```python
from build123d import *

# Parameters (mm, degrees)
F1_W            = 3.9823013358
F1_H            = 8.4623899311
F3_ANGLE_BACK   = 15
F3_ANGLE        = 30
F3_COPIES_COUNT = 4
F5_ANGLE_BACK   = 15
F5_ANGLE        = 30
F5_COPIES_COUNT = 4


# Not quite as in the source:
# - a pattern or mirror of a feature is missing from the dataset's text; its kind, count and spacing are read off the source's solid


with BuildPart() as f2:
    # F0 (on Front) → F2 (revolve)
    with BuildSketch(Plane.XZ):
        Polygon((0, 57.2826008411), (0, -18.7173991589), (18, -18.7173991589), (12.58260943, -15.5477793887), (8.3016352728, -13.0588412285), (8.3016352728, -4.7955662012), (8.3016352728, 1.6756732948), (8.3016352728, 5.1601859741), (9.1348709539, 7.4490089901), (10.7923932374, 10.6456615031), (10.7923932374, 16.8021768332), (8.3016352728, 20.8275895566), (8.3016352728, 28.1680505723), (9.7421156242, 29.4479895383), (8.7946596922, 30.5142838619), (9.8650568815, 31.4653853958), (8.8950488368, 32.5570605196), (9.914630721, 33.4630101088), (8.9067585183, 34.5972986517), (9.9263404025, 35.5032482409), (8.9067585183, 36.6507151981), (12.6114161685, 41.0112217069), (12.6114161685, 42.9367274046), (8.3016352728, 42.9367274046), (12.4439811334, 47.2063235939), (5.8302935213, 43.1041605771), (5.8302935213, 49.299262464), align=None)
    revolve(axis=Axis((0, 0, 19.2826008411), (0, 0, -1)))

    # F1 (on Front) → F3 (revolve)
    with BuildSketch(Plane.XZ, mode=Mode.PRIVATE) as f3_sk:
        with Locations((9.1009729076, 32.2875799611)):
            Rectangle(F1_W, F1_H)
    f3 = revolve(f3_sk.sketch.rotate(Axis((0, 0, 30.8512914926), (0, 0, -1)), -F3_ANGLE_BACK), axis=Axis((0, 0, 30.8512914926), (0, 0, -1)), revolution_arc=F3_ANGLE)

    # F3_copies: F3 ×4 about axis
    f3_copies_axis = Axis((0, 0, 0), (0, 0, 1))
    for i in range(1, F3_COPIES_COUNT):
        add(f3.rotate(f3_copies_axis, i * 360 / F3_COPIES_COUNT))

    # F4 (on Front) → F5 (revolve)
    with BuildSketch(Plane.XZ, mode=Mode.PRIVATE) as f5_sk:
        Polygon((8.193298243, 24.9484814703), (11.3307544962, 28.381921351), (8.193298243, 28.5003166646), align=None)
    f5 = revolve(f5_sk.sketch.rotate(Axis((0, 0, 30.8512914926), (0, 0, -1)), -F5_ANGLE_BACK), axis=Axis((0, 0, 30.8512914926), (0, 0, -1)), revolution_arc=F5_ANGLE)

    # F5_copies: F5 ×4 about axis
    f5_copies_axis = Axis((0, 0, 0), (0, 0, 1))
    for i in range(1, F5_COPIES_COUNT):
        add(f5.rotate(f5_copies_axis, i * 360 / F5_COPIES_COUNT))


solid = f2.part
```
Geometry: final body of the model. Coordinates: model frame, mm. A direction names the side the tool comes from. Give positions to 0.01 mm unless a question says otherwise; leave off trailing zeros. Order: outer loops, then holes, each group sorted by start corner. A loop starts at its lowest first (then second) coordinate and runs counter-clockwise, first axis right, second up. Notation, with made-up numbers: M -27,22.5 L 15,22.5 A14 cw 15,43.5 Z; hole C 15,73.25 d5. An arc over 180 degrees is marked long. Answer as CSV lines item,"result". Start each with the question number.
1) Set-up query: faces 1 (the cylindrical face through (0.041, -11.092, 32.512)), 2 (the flat face through (-2.535, -9.461, 30.873)), 3 (the flat face through (-9.461, 2.535, 30.873)). Return all of +Z, -Z, +X, -X, +Y, -Y with unobstructed straight access to the full face (end or side cutting, diameter ignored); none if empty.
2) First-contact query: P1, Ø2.5, axis at x = 0.5, y = 10, coming from the +Z side; P2, Ø3, axis at y = 1.5, z = 11, coming from the -X side; P3, Ø3, axis at x = 6.5, y = -9.5, coming from the +Z side. Flat tips, straight axial feed; report the tip coordinate or a pass-through.
3) Cut plane A-A (z = 12). Output: boundary loops of the cut face in (x, y).
4) Line query: line 1 (X direction, y = -8.5, z = 47); line 2 (Z direction, x = -4.5, y = 10); line 3 (X direction, y = 1.5, z = -5.5) (3 decimals). Output: solid intervals per line, ascending. Write a range as from..to.
5) Cut plane B-B (z = -8.5). Output: boundary loops of the cut face in (x, y).
Findings below:
1,face 1,"-Y"
1,face 2,"-X"
1,face 3,"+Y"
2,P1,"stops at z = 46.47"
2,P2,"stops at x = -10.79"
2,P3,"stops at z = 47.21"
3,outline,"C 0,0 d21.58"
4,line 1,"x = -8.81..-8.63, 8.63..8.81"
4,line 2,"z = -18.72..-14.61, 39.07..42.94, 45.68..46.29"
4,line 3,"x = -8.165..8.165"
5,outline,"C 0,0 d16.6"
